Design review of the part built by this model. Coordinates are the model's own, in mm. Face numbers are marked on the shaded views. A direction names the side the tool comes from. Coordinates: 2 decimals unless noted, no trailing zeros. Write each loop counter-clockwise with the first axis right and the second up, starting at its lowest first coordinate (ties: lowest second). Pieces come first, ordered by that corner, then holes.
Q1. For the marked faces 1 and 2, list the 3-axis set-ups (+Z, -Z, +X, -X, +Y, -Y) from which the entire face can be reached by the end or side of a thin tool; tool diameter is ignored.
Q2. Take a section at C-C, the plane z = 745. Write out the cut boundary in (x, y), plus the area to 3 significant figures.
Q3. Take a section at B-B, the plane x = -81. Write out the cut boundary in (y, z).
Q4. Take a section at A-A, the plane y = -373. Write out the cut boundary in (x, z).
Q5. Take a section at D-D, the plane y = -67. Write out the cut boundary in (x, z).
Q6. For L1, parallel to X at y = 108, z = 437.5; L2, parallel to Z at x = 40.5, y = -141; L3, parallel to Z at x = -148, y = -150.5, list the stretches that pass through material, from the lowest coordinate up.
Q7. For pin 1 Ø6 at (x, z) = (151.5, 491.5) entering from -Y; pin 2 Ø5 at (y, z) = (88.5, 214.5) entering from -X; pin 3 Ø8 at (x, z) = (-208.5, 458) entering from -Y, all flat-tipped, find the tip position at first contact; note any pin that passes through.
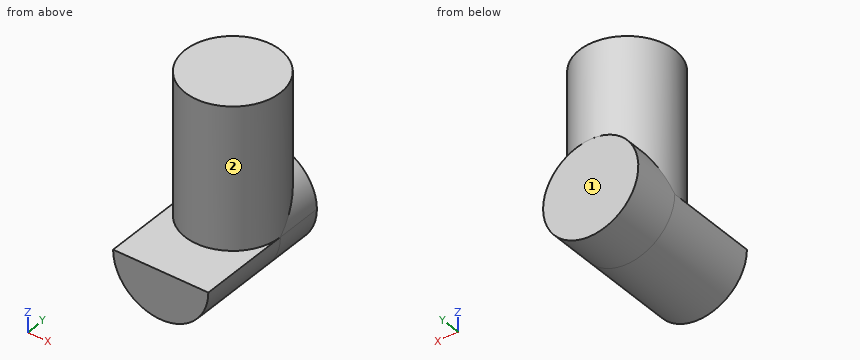
from build123d import *

# Parameters (mm, degrees)
F0_R     = 285.75
F1_DEPTH = 850.9
F2_R     = 285.75
F3_DEPTH = 285.75
F4_DEPTH = 565.15


with BuildPart() as f1:
    # F0 (on Top) → F1 (new body)
    with BuildSketch(Plane.XY):
        Circle(F0_R)
    extrude(amount=F1_DEPTH)

    # F2 (on Front) → F3 (join)
    with BuildSketch(Plane.XZ):
        Circle(F2_R)
    extrude(amount=-F3_DEPTH)

    # F3_face (on face) → F4 (join)
    with BuildSketch(Plane(origin=(0, 0, -121.276067), x_dir=(1, 0, 0), z_dir=(0, -1, 0))):
        with BuildLine():
            ThreePointArc((-285.75, 121.276067), (0, -164.473933), (285.75, 121.276067))
            Line((285.75, 121.276067), (-285.75, 121.276067))
        make_face()
    extrude(amount=F4_DEPTH)


solid = f1.part
Responses:
1. face 1: +Z, -Z, +X, -X, +Y
1. face 2: +Z
2. outline: circle Ø571.5 at (0, 0)
2. area: 257,000 mm2
3. outline: (-565.15, -274.03) - (285.75, -274.03) - (285.75, 274.03) - (274.03, 274.03) - (274.03, 850.9) - (-274.03, 850.9) - (-274.03, 0) - (-565.15, 0) - close
4. outline: (-285.75, 0) arc R285.75 ccw to (285.75, 0) - close
5. outline: (-285.75, 0) arc R285.75 ccw to (285.75, 0) - (277.78, 0) - (277.78, 850.9) - (-277.78, 850.9) - (-277.78, 0) - close
6. L1: x = -264.55 to 264.55
6. L2: z = -282.87 to 850.9
6. L3: z = -244.44 to 850.9
7. pin 1: stops at y = -244.13
7. pin 2: stops at x = -272.5
7. pin 3: stops at y = -199.58
